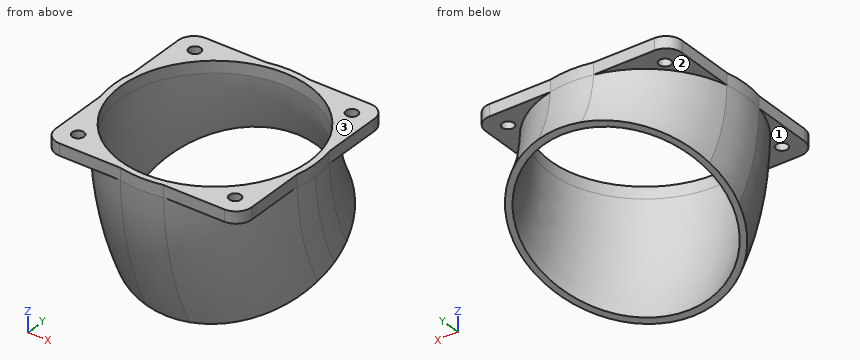
Autodesk Inventor part; units mm, degrees
ref_plane "YZ Plane" through (0, 0, 0) normal (1, 0, 0) x (0, 1, 0)
ref_plane "XZ Plane" through (0, 0, 0) normal (0, 1, 0) x (-1, 0, 0)
ref_plane "XY Plane" through (0, 0, 0) normal (0, 0, 1) x (1, 0, 0)
sketch "Szkic1" plane through (0, 0, 0) normal (0, 0, 1) x (1, 0, 0)
  circle A0 centre (0, 0) radius 24
  circle A1 centre (0, 0) radius 25.6
  line L0 (-21, 25) -> (-5.51, 25)
  line L1 (5.51, 25) -> (21, 25)
  line L2 (-25, -21) -> (-25, -5.51)
  line L3 (-25, 5.51) -> (-25, 21)
  line L4 (25, 21) -> (25, 5.51)
  line L5 (25, -5.51) -> (25, -21)
  line L6 (21, -25) -> (5.51, -25)
  line L7 (-5.51, -25) -> (-21, -25)
  arc A2 (-21, 25) -> (-25, 21) centre (-21, 21) ccw
  arc A3 (25, 21) -> (21, 25) centre (21, 21) ccw
  arc A4 (21, -25) -> (25, -21) centre (21, -21) ccw
  arc A5 (-25, -21) -> (-21, -25) centre (-21, -21) ccw
  point P0 (-25, 25)
  point P1 (25, -25)
  point P2 (25, 25)
  point P3 (-20, 20)
  point P4 (20, 20)
  point P5 (-20, -20)
  point P6 (20, -20)
  dimension "d0" = 48
  dimension "d1" = 50
  dimension "d2" = 50
  dimension "d5" = 40
  dimension "d6" = 40
  dimension "d7" = 20
  dimension "d8" = 20
  dimension "d9" = 1.6
  dimension "d10" = 4
sketch "Szkic2" plane through (0, 0, 0) normal (1, 0, 0) x (0, 1, 0)
  arc A0 (0, 0) -> (6.4705, -24.1481) centre (57.5642, 2.4833) ccw
  line L0 (0, 0) -> (6.4705, -24.1481) construction
  line L1 (0, 0) -> (25, 0) construction
  dimension "d11" = 25
  dimension "d12" = 75
sweep "Przeciągnięcie1" add profiles "Szkic1" path "Szkic2" contours A1
extrude "Wyciągnięcie proste1" add sketch "Szkic1" along normal blind 3
hole "Otwór1" at (-20, 20, 0) at (20, 20, 0) at (-20, -20, 0) at (20, -20, 0) direction (0, 0, 1) diameter 3 end through all
properties part number "3DP_ABS_Electronics_Colling_Tunnel"
Geometry check sheet. Reference: the model listing, model coordinates, mm. Face numbers are marked on the shaded views. Coordinates: 2 decimals unless noted, no trailing zeros.
Item 1: Release check for a two-part mould opening along Z. For the marked faces 1, 2 and 3 record: released by +Z, released by -Z, zero draft, split by the parting line, or undercut.
Item 2: Sectioned sample at A-A, the plane x = -20. Count the separate pieces of the cut face and the enclosed holes in it, then the cut area to 3 significant figures.
Item 3: Thickness scan on line 1 (Y direction, x = -20, z = 1.7); line 2 (X direction, y = 0, z = 2.25). Record the ranges inside material, lowest first.
Item 4: Go/stop test with flat-tipped pins: pin 1 Ø1 at (x, z) = (-8, -29.5) entering from -Y; pin 2 Ø2 at (x, z) = (-20.5, -14.5) entering from -Y; pin 3 Ø3.5 at (x, z) = (14.5, 2) entering from -Y. Record where each tip stops, or that it passes through.
Check result:
1. face 1: released by -Z
1. face 2: undercut
1. face 3: released by +Z
2. separate pieces: 4
2. enclosed holes: 0
2. area: 189 mm2
3. line 1: y = -25 to -21.5, -18.5 to -13.27, 13.27 to 18.5, 21.5 to 25
3. line 2: x = -25.6 to -24, 24 to 25.6
4. pin 1: stops at y = -18.13
4. pin 2: stops at y = -14.68
4. pin 3: stops at y = -25
